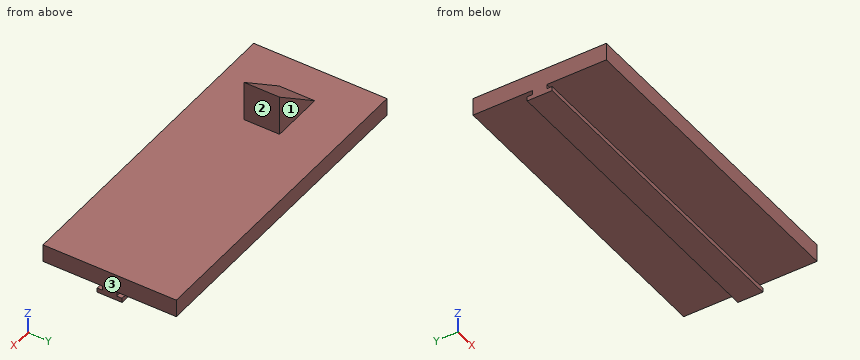
```python
from build123d import *

# Parameters (mm, degrees)
SKETCH1_W                = 457.2
SKETCH1_H                = 190.5
BOSS_EXTRUDE1_DEPTH      = 25.4
SKETCH2_W                = 457.2
SKETCH2_H                = 20.32
BOSS_EXTRUDE2_DEPTH      = 12.7
BOSS_EXTRUDE3_DEPTH      = 7.62
BOSS_EXTRUDE3_DEPTH_BACK = 27.94
SKETCH3_W                = 457.2
SKETCH3_H                = 6.35
BOSS_EXTRUDE5_DEPTH      = 25.4
BOSS_EXTRUDE5_DEPTH_BACK = 25.4


with BuildPart() as part:
    # Sketch1 → Boss-Extrude1 (new body)
    with BuildSketch(Plane.XY):
        Rectangle(SKETCH1_W, SKETCH1_H)
    extrude(amount=BOSS_EXTRUDE1_DEPTH)

    # Sketch2 → Boss-Extrude2 (add)
    with BuildSketch(Plane(origin=(0, 0, 0), x_dir=(-1, 0, 0), z_dir=(0, 0, -1))):
        Rectangle(SKETCH2_W, SKETCH2_H)
    extrude(amount=BOSS_EXTRUDE2_DEPTH)

    # Sketch3 → Boss-Extrude3 (add, two sides: drawn at the far end of the back side and taken through both)
    with BuildSketch(Plane(origin=(0, 10.16, 0), x_dir=(1, 0, 0), z_dir=(0, 1, 0)).offset(-BOSS_EXTRUDE3_DEPTH_BACK)):
        with Locations((0, 9.525)):
            Rectangle(SKETCH3_W, SKETCH3_H)
    extrude(amount=BOSS_EXTRUDE3_DEPTH + BOSS_EXTRUDE3_DEPTH_BACK)

    # Sketch5 → Boss-Extrude5 (add, two sides: drawn at the far end of the back side and taken through both)
    with BuildSketch(Plane(origin=(0, 0, 0), x_dir=(1, 0, 0), z_dir=(0, 1, 0)).offset(-BOSS_EXTRUDE5_DEPTH_BACK)):
        Polygon((-177.8, -25.4), (-101.6, -25.4), (-101.6, -82.55), align=None)
    extrude(amount=BOSS_EXTRUDE5_DEPTH + BOSS_EXTRUDE5_DEPTH_BACK)


solid = part.part
```
Check sheet for the modelled part. Datum: model origin and axes. Units: mm. Face numbers are marked on the shaded views. A direction names the side the tool comes from. Round coordinates to 2 decimals unless told otherwise and drop trailing zeros. Order: outer loops, then holes, each group sorted by start corner. A loop starts at its lowest first (then second) coordinate and runs counter-clockwise, first axis right, second up. Notation, with made-up numbers: M 7,16.5 L 66,16.5 A26 cw 66,39.5 Z; hole C 88,-10.5 d9. An arc over 180 degrees is marked long. Answer in a Markdown table with one row per item.
(1) Section check D-D on x = -134.5. Record the boundary of the cut face in (y, z) (3 decimals).
Findings:
| item | result |
|---|---|
| outline | M -95.25,0 L -10.16,0 L -10.16,-6.35 L -17.78,-6.35 L -17.78,-12.7 L 17.78,-12.7 L 17.78,-6.35 L 10.16,-6.35 L 10.16,0 L 95.25,0 L 95.25,25.4 L 25.4,25.4 L 25.4,57.875 L -25.4,57.875 L -25.4,25.4 L -95.25,25.4 Z |
(2) Material ranges on line 1 along Z through (x, y) = (66.5, -11.5); line 2 along Z through (x, y) = (-13.5, -84.5); line 3 along Z through (x, y) = (-90.5, 8), recorded low to high. Write a range as from..to.
Findings:
| item | result |
|---|---|
| line 1 | z = -12.7..-6.35, 0..25.4 |
| line 2 | z = 0..25.4 |
| line 3 | z = -12.7..25.4 |
(3) Gauge pin test, flat ends, axial feed: pin 1 (6 mm diameter, centred on x = -96, y = -13, fed in from +Z); pin 2 (3 mm diameter, centred on x = -99, z = -9.5, fed in from -Y); pin 3 (5 mm diameter, centred on x = 61, z = -8.5, fed in from +Y). Record the tip position at first contact, or that the pin passes through.
Findings:
| item | result |
|---|---|
| pin 1 | stops at z = 25.4 |
| pin 2 | stops at y = -17.78 |
| pin 3 | stops at y = 17.78 |
(4) Section check C-C on z = 72.5. Record the boundary of the cut face in (x, y).
Findings:
| item | result |
|---|---|
| outline | M -115,-25.4 L -101.6,-25.4 L -101.6,25.4 L -115,25.4 Z |
(5) Section check A-A on x = 29. Record the boundary of the cut face in (y, z), plus the area to 3 significant figures.
Findings:
| item | result |
|---|---|
| outline | M -95.25,0 L -10.16,0 L -10.16,-6.35 L -17.78,-6.35 L -17.78,-12.7 L 17.78,-12.7 L 17.78,-6.35 L 10.16,-6.35 L 10.16,0 L 95.25,0 L 95.25,25.4 L -95.25,25.4 Z |
| area | 5,190 mm^2 |
(6) Section check B-B on y = 0. Record the boundary of the cut face in (x, z).
Findings:
| item | result |
|---|---|
| outline | M -228.6,-12.7 L 228.6,-12.7 L 228.6,25.4 L -101.6,25.4 L -101.6,82.55 L -177.8,25.4 L -228.6,25.4 Z |
(7) Set-up check for the marked faces 1, 2 and 3: record each of +Z, -Z, +X, -X, +Y, -Y from which the full face is reachable in a straight line by a thin tool's end or side.
Findings:
| item | result |
|---|---|
| face 1 | +Z, +X, -X, +Y |
| face 2 | +Z, +X, +Y, -Y |
| face 3 | +Z, -Z, +X, +Y, -Y |
